```python
from build123d import *

# Parameters (mm, degrees)
SKETCH_2_OUTSIDE_W   = 51.54
SKETCH_2_OUTSIDE_H   = 51.54
SKETCH_2_OUTSIDE_W_2 = 13.7
SKETCH_2_OUTSIDE_H_2 = 13.7
CUT_EXTRUDE_1_DEPTH  = 16.5
CHAMFER_1_SIZE       = 1


with BuildPart() as part:
    # 草图1 → 旋转1 (revolve)
    with BuildSketch(Plane(origin=(0, 0, 0), x_dir=(0, 0, -1), z_dir=(1, 0, 0)), mode=Mode.PRIVATE) as revolve_1_sk:
        Polygon((-117.5, 0), (0, 0), (0, 5), (-20, 5), (-20, 9), (-36.5, 9), (-36.5, 12.5), (-39.5, 12.5), (-39.5, 10), (-64.5, 10), (-64.5, 9), (-67.5, 9), (-67.5, 10), (-117.5, 10), align=None)
    revolve(revolve_1_sk.sketch.rotate(Axis((0, 0, 117.5), (0, 0, -1)), 90), axis=Axis((0, 0, 117.5), (0, 0, -1)))

    # 草图2 outside → 切除-拉伸1 (cut)
    with BuildSketch(Plane(origin=(0, 0, 20), x_dir=(-1, 0, 0), z_dir=(0, 0, -1))):
        Rectangle(SKETCH_2_OUTSIDE_W, SKETCH_2_OUTSIDE_H)
        Rectangle(SKETCH_2_OUTSIDE_W_2, SKETCH_2_OUTSIDE_H_2, mode=Mode.SUBTRACT)
    extrude(amount=-CUT_EXTRUDE_1_DEPTH, mode=Mode.SUBTRACT)

    # 倒角1
    chamfer_1_edges = [part.edges().sort_by_distance(p)[0] for p in [
        (-5, 0, 0),
        (-10, 0, 117.5),
    ]]
    chamfer(chamfer_1_edges, length=CHAMFER_1_SIZE)


solid = part.part
```
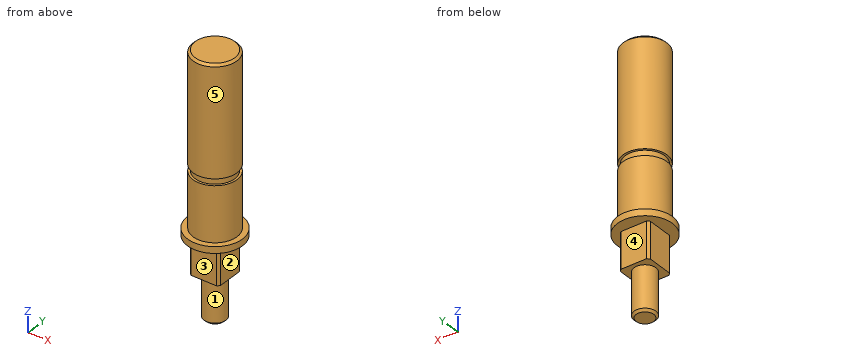
The listing builds one solid part. Answer for the finished solid, in the listing's coordinates (mm). Face numbers are marked on the shaded views. A direction names the side the tool comes from. Round coordinates to 2 decimals unless told otherwise and drop trailing zeros. Write each loop counter-clockwise with the first axis right and the second up, starting at its lowest first coordinate (ties: lowest second). Pieces come first, ordered by that corner, then holes. Notation, with made-up numbers: (8, 13) -> (14, 13) arc R10 cw to (14, 18) -> close; hole circle Ø7 at (-26, -9). An arc over 180 degrees is marked (long way). Write item = value, one per line.
1) Section D-D on z = 62.5 is taken. Write down the section's boundary in (x, y), plus the area to 3 significant figures.
Check values:
outline = circle Ø20 at (0, 0)
area = 314 mm²
2) Which of the six approach directions +Z, -Z, +X, -X, +Y, -Y give full straight-line access (tool end or side, diameter ignored) to the marked faces 1, 2, 3, 4 and 5?
Check values:
face_1 = -Z
face_2 = -Z, +X, +Y, -Y
face_3 = -Z, +X, -X, -Y
face_4 = -Z, +X, -X, +Y
face_5 = +Z
3) Given pin 1 (11 mm diameter, centred on x = 1.5, y = 0.5, fed in from -Z); pin 2 (9.5 mm diameter, centred on y = -1.5, z = 25.5, fed in from +X); pin 3 (12 mm diameter, centred on x = -10, y = 7.5, fed in from -Z); pin 4 (9.5 mm diameter, centred on x = -0.5, z = 28, fed in from +Y), each flat-ended and moving along its own axis, determine where each tip first touches the part or whether it passes through.
Check values:
pin_1 = 0
pin_2 = 6.85
pin_3 = 20
pin_4 = 6.85
4) Straight lines are drawn through the part: line 1 along Z through (x, y) = (0.25, -8.75); line 2 along Z through (x, y) = (-9.25, -1.25); line 3 along Z through (x, y) = (-7.75, -9.75). For each, find the intervals that lie inside material, in ascending order. Write a range as [from, to].
Check values:
line_1 = [36.5, 117.5]
line_2 = [36.5, 64.5], [67.5, 117.17]
line_3 = [36.5, 39.5]
5) Section A-A on z = 25.5 is taken. Write down the section's boundary in (x, y).
Check values:
outline = (-6.85, -5.84) arc R9 ccw to (-5.84, -6.85) -> (5.84, -6.85) arc R9 ccw to (6.85, -5.84) -> (6.85, 5.84) arc R9 ccw to (5.84, 6.85) -> (-5.84, 6.85) arc R9 ccw to (-6.85, 5.84) -> close
6) Section B-B on y = 0 is taken. Write down the section's boundary in (x, z).
Check values:
outline = (-12.5, 36.5) -> (-6.85, 36.5) -> (-6.85, 20) -> (-5, 20) -> (-5, 1) -> (-4, 0) -> (4, 0) -> (5, 1) -> (5, 20) -> (6.85, 20) -> (6.85, 36.5) -> (12.5, 36.5) -> (12.5, 39.5) -> (10, 39.5) -> (10, 64.5) -> (9, 64.5) -> (9, 67.5) -> (10, 67.5) -> (10, 116.5) -> (9, 117.5) -> (-9, 117.5) -> (-10, 116.5) -> (-10, 67.5) -> (-9, 67.5) -> (-9, 64.5) -> (-10, 64.5) -> (-10, 39.5) -> (-12.5, 39.5) -> close
